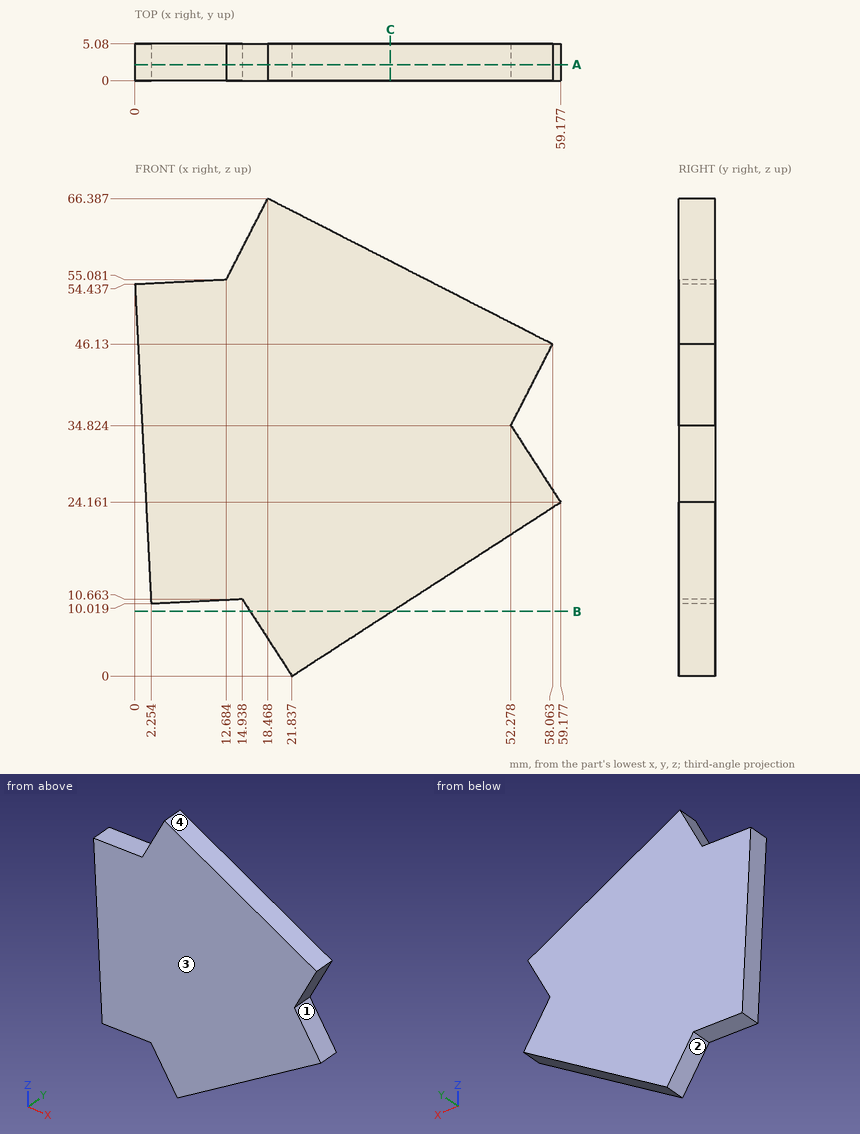
Geometry check sheet. Reference: drawing and pictorial views, mm from the part's lowest x, y, z. Coordinates: 2 decimals unless noted, no trailing zeros. Write each loop counter-clockwise with the first axis right and the second up, starting at its lowest first coordinate (ties: lowest second). Pieces come first, ordered by that corner, then holes. Notation, with made-up numbers: M -23.5,69 L 34.5,69 A17 ccw 34.5,77 Z; hole C -19.75,74 d6. An arc over 180 degrees is marked long. Write item = value, one per line. Start each with the question number.
1. Thickness scan on probe 1 along Z at (x, y) = (28, 1.1); probe 2 along Z at (x, y) = (15, 4.65) (1 decimal); probe 3 along X at (y, z) = (0.25, 36) (1 decimal). Record the ranges inside material, lowest first.
2. Sectioned sample at A-A (y = 2.2). Record the cut outline in (x, z).
3. Mould release check, pull along Z, two halves, no side actions. Record for the marked faces 1, 2, 3 and 4: pulls with the +Z half, pulls with the -Z half, needs draft (parallel to the pull), parting line crosses it, or undercut.
4. Sectioned sample at C-C (x = 35.5). Record the cut outline in (y, z), then the cut area to 3 significant figures.
5. Go/stop test with flat-tipped pins: pin 1 (5 mm diameter, centred on x = 38, z = 38, fed in from -Y); pin 2 (1.5 mm diameter, centred on x = 42.5, y = 1, fed in from -Z) (1 decimal); pin 3 (1 mm diameter, centred on y = 4, z = 48, fed in from -X). Record where each tip stops, or that it passes through.
6. Sectioned sample at B-B (z = 9). Record the cut outline in (x, y), then the cut area to 3 significant figures.
The answers:
q1.probe_1 = 3.99 to 61.51
q1.probe_2 = 10.6 to 59.6
q1.probe_3 = 0.9 to 52.9
q2.outline = M 0,54.44 L 2.25,10.02 L 14.94,10.66 L 21.84,0 L 59.18,24.16 L 52.28,34.82 L 58.06,46.13 L 18.47,66.39 L 12.68,55.08 Z
q3.face_1 = undercut
q3.face_2 = pulls with the -Z half
q3.face_3 = needs draft
q3.face_4 = pulls with the +Z half
q4.outline = M 0,8.84 L 5.08,8.84 L 5.08,57.67 L 0,57.67 Z
q4.area = 248 mm²
q5.pin_1 = 0
q5.pin_2 = 12.9
q5.pin_3 = 0.3
q6.outline = M 16.01,0 L 35.75,0 L 35.75,5.08 L 16.01,5.08 Z
q6.area = 100 mm²
